```python
from build123d import *

# Parameters (mm, degrees)
SKETCH_1_W          = 138
SKETCH_1_H          = 65.6
SKETCH_1_R          = 1.4
EXTRUDE_1_DEPTH     = 2
SKETCH_2_W          = 138
SKETCH_2_H          = 32.6
EXTRUDE_2_DEPTH     = 5
SKETCH_3_W          = 138
SKETCH_3_H          = 2
EXTRUDE_3_DEPTH     = 45
FILLET_1_R          = 10
SKETCH_5_W          = 138
SKETCH_5_H          = 2
EXTRUDE_4_DEPTH     = 15
FILLET_2_R          = 10
CUT_EXTRUDE_1_REACH = 90.667
SKETCH_6_W          = 15
SKETCH_6_H          = 25.6
FILLET_3_R          = 1
FILLET_4_R          = 1


with BuildPart() as part:
    # 草图1 → 凸台-拉伸1 (new body)
    with BuildSketch(Plane(origin=(0, 0, 0), x_dir=(1, 0, 0), z_dir=(0, 1, 0))):
        Rectangle(SKETCH_1_W, SKETCH_1_H)
        with Locations(Location((-64, 9.8, 0), (0, 0, 270))):
            Circle(SKETCH_1_R, mode=Mode.SUBTRACT)
        with Locations(Location((64, 9.8, 0), (0, 0, 270))):
            Circle(SKETCH_1_R, mode=Mode.SUBTRACT)
    extrude(amount=EXTRUDE_1_DEPTH)

    # 草图2 → 凸台-拉伸2 (add)
    with BuildSketch(Plane(origin=(0, 2, 0), x_dir=(1, 0, 0), z_dir=(0, 1, 0))):
        with Locations((0, -16.5)):
            Rectangle(SKETCH_2_W, SKETCH_2_H)
    extrude(amount=EXTRUDE_2_DEPTH)

    # 草图3 → 凸台-拉伸3 (add)
    with BuildSketch(Plane.XZ):
        with Locations((0, -31.8)):
            Rectangle(SKETCH_3_W, SKETCH_3_H)
    extrude(amount=EXTRUDE_3_DEPTH)

    # 圆角1
    fillet_1_edges = [part.edges().sort_by_distance(p)[0] for p in [
        (-69, 4.5, 0.2),
        (69, 4.5, 0.2),
    ]]
    fillet(fillet_1_edges, radius=FILLET_1_R)

    # 草图5 → 凸台-拉伸4 (add)
    with BuildSketch(Plane.XZ):
        with Locations((0, 31.8)):
            Rectangle(SKETCH_5_W, SKETCH_5_H)
    extrude(amount=EXTRUDE_4_DEPTH)

    # 圆角2
    fillet_2_edges = [part.edges().sort_by_distance(p)[0] for p in [
        (-69, -45, -31.8),
        (69, -45, -31.8),
        (-69, -15, 31.8),
        (69, -15, 31.8),
    ]]
    fillet(fillet_2_edges, radius=FILLET_2_R)

    # 切除-拉伸1: up to this face of the body (flat: up to its plane)
    cut_extrude_1_end = Plane(part.part.faces().sort_by_distance((0, 7, 16.635491013))[0])
    # 草图6 → 切除-拉伸1 (cut, up to the picked face)
    with BuildSketch(Plane.XZ, mode=Mode.PRIVATE) as cut_extrude_1_sk1:
        with Locations((-51.5, 13)):
            Rectangle(SKETCH_6_W, SKETCH_6_H)
    cut_extrude_1_tool1 = split(extrude(cut_extrude_1_sk1.sketch, amount=-CUT_EXTRUDE_1_REACH, mode=Mode.PRIVATE), bisect_by=cut_extrude_1_end, keep=Keep.BOTH, mode=Mode.PRIVATE)
    # 草图6 → 切除-拉伸1 (cut, up to the picked face)
    with BuildSketch(Plane.XZ, mode=Mode.PRIVATE) as cut_extrude_1_sk2:
        with Locations((51.5, 13)):
            Rectangle(SKETCH_6_W, SKETCH_6_H)
    cut_extrude_1_tool2 = split(extrude(cut_extrude_1_sk2.sketch, amount=-CUT_EXTRUDE_1_REACH, mode=Mode.PRIVATE), bisect_by=cut_extrude_1_end, keep=Keep.BOTH, mode=Mode.PRIVATE)
    add(cut_extrude_1_tool1.solids().sort_by(Axis((-51.5, 0, 13), (0, 1, 0)))[0], mode=Mode.SUBTRACT)
    add(cut_extrude_1_tool2.solids().sort_by(Axis((51.5, 0, 13), (0, 1, 0)))[0], mode=Mode.SUBTRACT)

    # 圆角3
    fillet_3_edges = [part.edges().sort_by_distance(p)[0] for p in [
        (-59, 3.5, 25.8),
        (-44, 3.5, 25.8),
        (59, 3.5, 25.8),
        (44, 3.5, 25.8),
    ]]
    fillet(fillet_3_edges, radius=FILLET_3_R)

    # 圆角4
    fillet_4_edges = [part.edges().sort_by_distance(p)[0] for p in [
        (-44, 1, 0.2),
        (-59, 1, 0.2),
        (59, 1, 0.2),
        (44, 1, 0.2),
    ]]
    fillet(fillet_4_edges, radius=FILLET_4_R)


solid = part.part
```
For this review, take the finished solid that the model builds, in its own axes (mm). A direction names the side the tool comes from. Coordinates: 2 decimals unless noted, no trailing zeros. Order: outer loops, then holes, each group sorted by start corner. A loop starts at its lowest first (then second) coordinate and runs counter-clockwise, first axis right, second up. Notation, with made-up numbers: (34.25, 38) - (61.25, 38) arc R10 cw to (61.25, 46) - close; hole circle Ø7 at (21.5, -30.75). An arc over 180 degrees is marked (long way). Answer as a JSON object with one key per item and string values. Group by question number.
1. The part is to be moulded in two halves that separate along Z. For faces 5 (the cylindrical face through (-66.15, 4.54, 3.21)), 6 (the flat face through (51, 3, 25.8)), 7 (the flat face through (-69, 1.7, -0.2)), 8 (the cylindrical face through (65.39, 0.99, -9.98)), say which applies: pulls with the +Z half, pulls with the -Z half, needs draft (parallel to the pull), parting line crosses it, or undercut.
2. For faces 1 (the flat face through (-1, 4, 0.2)), 2 (the cylindrical face through (66.15, -11.99, 31.81)), 3 (the flat face through (-52, 3, 25.8)), 4 (the flat face through (-1, -22, -30.8)), list the 3-axis set-ups (+Z, -Z, +X, -X, +Y, -Y) from which the entire face can be reached by the end or side of a thin tool; tool diameter is ignored.
3. Clearance check with flat-ended pins moving along their axes: P1, Ø10, axis at x = 19, y = -39.5, coming from the +Z side; P2, Ø4, axis at x = -6.5, y = 5, coming from the -Z side; P3, Ø3, axis at x = 64, z = -9.8, coming from the +Y side. State where each tip first meets the part, or that it passes through.
4. We need section D-D on y = -11.5. State the section outline as (x, z) points.
5. For probe 1 along X at (y, z) = (4.5, 25); probe 2 along X at (y, z) = (0.5, -9.8); probe 3 along Z at (x, y) = (64, 1.3), list the stretches that pass through material, from the lowest coordinate up.
6. We need section C-C on x = -64. State the section outline as (y, z) points, then the cut area to 3 significant figures.
7. We need section B-B on z = 23. State the section outline as (x, y) points, then the cut area to 3 significant figures.
8. We need section A-A on z = -9.8. State the section outline as (x, y) points, then the cut area to 3 significant figures.
Final values:
{
 "1": {"face 5": "pulls with the -Z half", "face 6": "undercut", "face 7": "needs draft", "face 8": "undercut"},
 "2": {"face 1": "-Z, +X, -X, +Y", "face 2": "+Z, +X, -Y", "face 3": "+Y, -Y", "face 4": "+X, -X, -Y"},
 "3": {"P1": "z = -30.8", "P2": "z = 0.2", "P3": "y = 2"},
 "4": {"outline": "(-69, -32.8) - (69, -32.8) - (69, -30.8) - (-69, -30.8) - close; (-66.6, 30.8) - (66.6, 30.8) - (66.6, 32.8) - (-66.6, 32.8) - close"},
 "5": {"probe 1": "-69 to -58.98, -44.02 to 44.02, 58.98 to 69", "probe 2": "-69 to -65.4, -62.6 to 62.6, 65.4 to 69", "probe 3": "-32.8 to -11.2, -8.4 to 32.8"},
 "6": {"outline": "(-43.66, -32.8) - (2, -32.8) - (2, -11.2) - (0, -11.2) - (0, -30.8) - (-43.66, -30.8) - close; (-13.66, 30.8) - (0, 30.8) - (0, -8.4) - (2, -8.4) - (2, 1.54) - (7, 1.54) - (7, 32.8) - (-13.66, 32.8) - close", "area": "397 mm²"},
 "7": {"outline": "(-69, 0) - (-59, 0) - (-59, 7) - (-69, 7) - close; (-44, 0) - (44, 0) - (44, 7) - (-44, 7) - close; (59, 0) - (69, 0) - (69, 7) - (59, 7) - close", "area": "756 mm²"},
 "8": {"outline": "(-69, 0) - (-65.4, 0) - (-65.4, 2) - (-69, 2) - close; (-62.6, 0) - (62.6, 0) - (62.6, 2) - (-62.6, 2) - close; (65.4, 0) - (69, 0) - (69, 2) - (65.4, 2) - close", "area": "265 mm²"}
}
